Geometry: final body of the model. Coordinates: model frame, mm. A direction names the side the tool comes from. Coordinates: 2 decimals unless noted, no trailing zeros. Loops run counter-clockwise (first coordinate to the right, second up) from the corner with the lowest first, then second, coordinate; pieces in that order, holes last. Notation, with made-up numbers: (53.5, 60) - (91.5, 60) arc R12 ccw to (91.5, 79) - close; hole circle Ø8 at (31.5, 3.25). An arc over 180 degrees is marked (long way). Answer in a Markdown table with one row per item.
from build123d import *

# Parameters (mm, degrees)
SKETCH1_R           = 4.05
BOSS_EXTRUDE1_DEPTH = 20
SKETCH3_R           = 2.65
CUT_EXTRUDE5_DEPTH  = 40
SKETCH6_R           = 5.5
CUT_EXTRUDE7_DEPTH  = 29
CHAMFER1_SIZE       = 2
FILLET1_R           = 1


with BuildPart() as part:
    # Sketch1 → Boss-Extrude1 (new body)
    with BuildSketch(Plane(origin=(0, 0, 0), x_dir=(1, 0, 0), z_dir=(0, 1, 0))):
        with BuildLine():
            Line((10, -20), (-20, -20))
            Line((-20, -20), (-20, 20))
            Line((-20, 20), (20, 20))
            Line((20, 20), (20, -10))
            ThreePointArc((20, -10), (17.071067812, -17.071067812), (10, -20))
        make_face()
        with Locations(Location((0, 0, 0), (0, 0, 270))):
            Circle(SKETCH1_R, mode=Mode.SUBTRACT)
    extrude(amount=BOSS_EXTRUDE1_DEPTH)

    # Sketch3 → Cut-Extrude5 (cut)
    with BuildSketch(Plane.XY.offset(20)):
        with Locations((-13, 10)):
            Circle(SKETCH3_R)
        with Locations((13, 10)):
            Circle(SKETCH3_R)
    extrude(amount=-CUT_EXTRUDE5_DEPTH, mode=Mode.SUBTRACT)

    # Sketch6 → Cut-Extrude7 (cut)
    with BuildSketch(Plane.XY.offset(20)):
        with Locations((-13, 10)):
            Circle(SKETCH6_R)
        with Locations((13, 10)):
            Circle(SKETCH6_R)
    extrude(amount=-CUT_EXTRUDE7_DEPTH, mode=Mode.SUBTRACT)

    # Chamfer1
    chamfer1_edges = [part.edges().sort_by_distance(p)[0] for p in [
        (17.071067812, 20, 17.071067812),
        (20, 20, -5),
        (-5, 20, 20),
    ]]
    chamfer(chamfer1_edges, length=CHAMFER1_SIZE)

    # Fillet1
    fillet1_edges = [part.edges().sort_by_distance(p)[0] for p in [
        (0, 20, -4.05),
    ]]
    fillet(fillet1_edges, radius=FILLET1_R)


solid = part.part
(1) Cut plane B-B on y = 18.5. Output: boundary loops of the cut face in (x, z).
Verdict:
| item | result |
|---|---|
| outline | (-20, -20) - (19.5, -20) - (19.5, 10) arc R9.5 ccw to (10, 19.5) - (-20, 19.5) - close; hole circle Ø8.1 at (0, 0) |
(2) Cut plane C-C on x = -13. Output: boundary loops of the cut face in (y, z), then the cut area to 3 significant figures.
Verdict:
| item | result |
|---|---|
| outline | (0, -20) - (7.35, -20) - (7.35, -9) - (4.5, -9) - (4.5, 20) - (0, 20) - close; (12.65, -20) - (20, -20) - (20, 18) - (18, 20) - (15.5, 20) - (15.5, -9) - (12.65, -9) - close |
| area | 421 mm² |
(3) Pull-direction query (Y, two-part tool) for faces 3 (the face through (-4.2, 0, -0.3)), 4 (the face through (7.505, 10.242, 5.703)), 5 (the face through (-5, 19, 19)), 6 (the face through (0, 10, -20)); classes: pulls with the +Y half, pulls with the -Y half, needs draft (parallel to the pull), parting line crosses it, or undercut.
Verdict:
| item | result |
|---|---|
| face 3 | pulls with the -Y half |
| face 4 | undercut |
| face 5 | pulls with the +Y half |
| face 6 | needs draft |
(4) Cut plane A-A on z = 0. Output: boundary loops of the cut face in (x, y), then the cut area to 3 significant figures.
Verdict:
| item | result |
|---|---|
| outline | (-20, 0) - (-4.05, 0) - (-4.05, 19) arc R1 ccw to (-5.05, 20) - (-20, 20) - close; (4.05, 0) - (20, 0) - (20, 18) - (18, 20) - (5.05, 20) arc R1 ccw to (4.05, 19) - close; hole circle Ø11 at (-13, 10); hole circle Ø11 at (13, 10) |
| area | 446 mm² |
(5) Cut plane D-D on z = -12.5. Output: boundary loops of the cut face in (x, y), then the cut area to 3 significant figures.
Verdict:
| item | result |
|---|---|
| outline | (-20, 0) - (20, 0) - (20, 18) - (18, 20) - (-20, 20) - close; hole circle Ø5.3 at (-13, 10); hole circle Ø5.3 at (13, 10) |
| area | 754 mm² |
(6) Access query for faces 1 (the face through (18, 7, 16)), 2 (the face through (-16, 9, -9)). Directions: +Z, -Z, +X, -X, +Y, -Y. A direction counts if a zero-diameter tool reaches every point of the face in a straight line with its end or side. Return the directions, or none.
Verdict:
| item | result |
|---|---|
| face 1 | +Z, +X, +Y, -Y |
| face 2 | +Z |
(7) First-contact query: pin 1 Ø5.5 at (x, y) = (14, 11) entering from +Z. Flat tip, straight axial feed; report the tip coordinate or a pass-through.
Verdict:
| item | result |
|---|---|
| pin 1 | stops at z = -9 |
(8) Ray query, probe 1 along X at (y, z) = (15, 13); probe 2 along Y at (x, z) = (13, -12.5); probe 3 along X at (y, z) = (10.75, 7). Return the intervals inside material, ascending.
Verdict:
| item | result |
|---|---|
| probe 1 | x = -20 to -15.29, -10.71 to 10.71, 15.29 to 19.54 |
| probe 2 | y = 0 to 7.35, 12.65 to 20 |
| probe 3 | x = -20 to -18.45, -7.55 to 7.55, 18.45 to 20 |
